Answer from the drawing. Dimensions are ordinates in mm from the lowest x, y and z of the part. Round coordinates to 2 decimals unless told otherwise and drop trailing zeros. Write each loop counter-clockwise with the first axis right and the second up, starting at its lowest first coordinate (ties: lowest second). Pieces come first, ordered by that corner, then holes. Notation, with made-up numbers: (58.5, 54.25) - (69.5, 54.25) arc R3 cw to (69.5, 59.25) - close; hole circle Ø3 at (-24.5, 32). An arc over 180 degrees is marked (long way). One line per item, written item: value. Start each with the question number.
(1) Find the intervals of material crossed by L1, parallel to Y at x = 11.5, z = 17; L2, parallel to Y at x = 10.75, z = 16.5; L3, parallel to X at y = 143, z = 11.75, in increasing order.
(2) A cutting plane is placed at C-C, the plane y = 130.5. Determine the outline of the cut face in (x, z), plus the area to 3 significant figures.
(3) A cutting plane is placed at D-D, the plane z = 1.5. Determine the outline of the cut face in (x, y).
(4) A cutting plane is placed at A-A, the plane x = 11.5. Determine the outline of the cut face in (y, z), plus the area to 3 significant figures.
(5) A cutting plane is placed at B-B, the plane z = 16. Determine the outline of the cut face in (x, y).
(6) Flat-ended cylindrical pins translate along their axes: pin 1 Ø0.9 at (x, y) = (11, 53) entering from +Z; pin 2 Ø8 at (x, y) = (4, 113) entering from -Z; pin 3 Ø3 at (x, y) = (8, 60) entering from -Z; pin 4 Ø10 at (x, y) = (16, 137.5) entering from -Z. Find the tip coordinate at first contact, or state that the pin passes through.
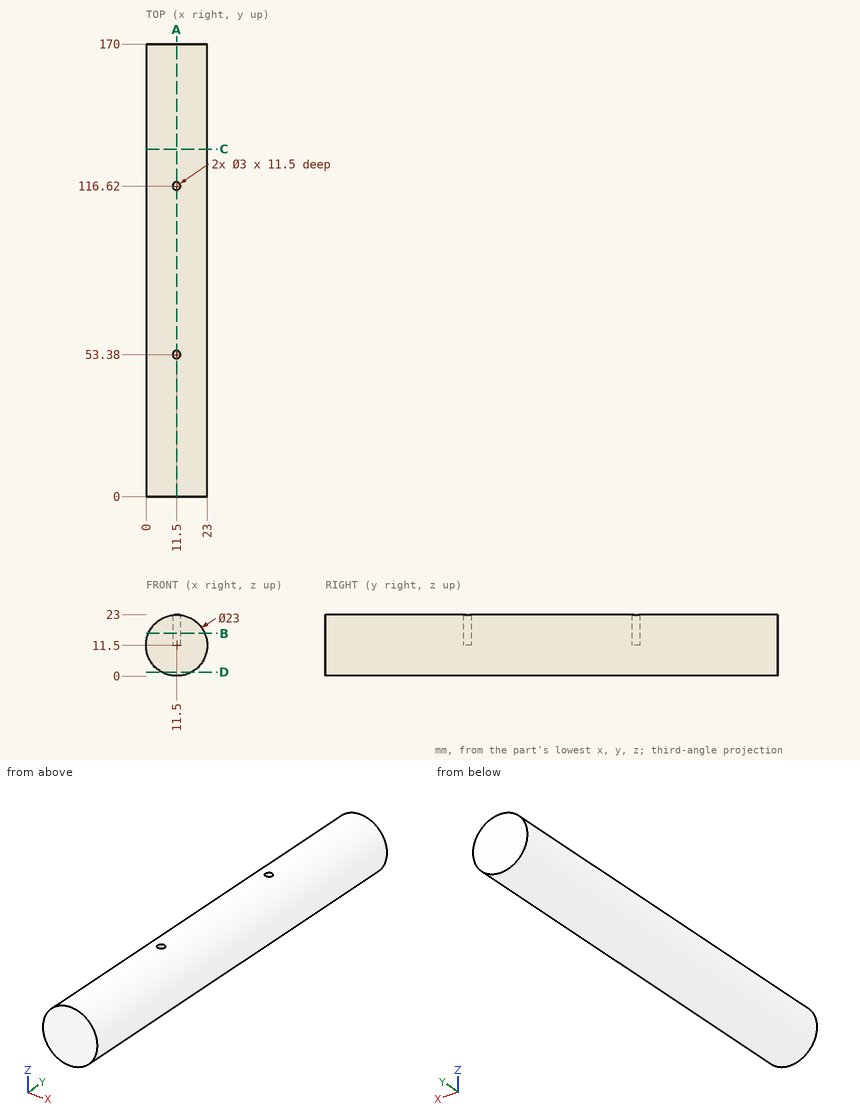
Here are the results:
1. L1: 0 to 51.88, 54.88 to 115.12, 118.12 to 170
1. L2: 0 to 52.08, 54.68 to 115.32, 117.92 to 170
1. L3: 0 to 23
2. outline: circle Ø23 at (11.5, 11.5)
2. area: 415 mm²
3. outline: (5.82, 0) - (17.18, 0) - (17.18, 170) - (5.82, 170) - close
4. outline: (0, 0) - (170, 0) - (170, 23) - (118.12, 23) - (118.12, 11.5) - (115.12, 11.5) - (115.12, 23) - (54.88, 23) - (54.88, 11.5) - (51.88, 11.5) - (51.88, 23) - (0, 23) - close
4. area: 3,840 mm²
5. outline: (0.92, 0) - (22.08, 0) - (22.08, 170) - (0.92, 170) - close; hole circle Ø3 at (11.5, 53.38); hole circle Ø3 at (11.5, 116.62)
6. pin 1: z = 11.5
6. pin 2: z = 0.55
6. pin 3: z = 0.18
6. pin 4: z = 0
